```python
from build123d import *

# Parameters (mm, degrees)
F0_W     = 14.0914916992
F0_H     = 13.3883208036
F0_H_2   = 4.0725544095
F1_DEPTH = 25.4
F2_R     = 5.08


with BuildPart() as f1:
    # F0 (on Top) → F1 (new body)
    with BuildSketch(Plane.XY):
        Polygon((-14.0914916992, 52.0800277591), (-14.0914916992, 65.4683485627), (0, 65.4683485627), (0, 52.0800277591), (26.658244431, 52.0800277591), (26.658244431, 110.8265519142), (-39.2834246159, 110.8265519142), (-39.2834246159, 52.0800277591), align=None)
        with Locations((-7.0457458496, 58.7741881609)):
            Rectangle(F0_W, F0_H)
        with Locations((-7.0457458496, 50.0437505543)):
            Rectangle(F0_W, F0_H_2)
    extrude(amount=F1_DEPTH)

    # F2
    f2_edges = [f1.edges().sort_by_distance(p)[0] for p in [
        (26.658244, 81.45329, 25.4),
        (26.658244, 81.45329, 0),
        (-39.283425, 81.45329, 25.4),
        (-6.31259, 110.826552, 25.4),
    ]]
    fillet(f2_edges, radius=F2_R)


solid = f1.part
```
Build history of the part. All positions in model axes, mm. A direction names the side the tool comes from. Coordinates: 2 decimals unless noted, no trailing zeros. Order: outer loops, then holes, each group sorted by start corner. A loop starts at its lowest first (then second) coordinate and runs counter-clockwise, first axis right, second up. Notation, with made-up numbers: M 2,16 L 24,16 A25 ccw 24,33 Z; hole C 66,-21.5 d11. An arc over 180 degrees is marked long. One line per question, with ' | ' between items. Start each with the question number.
1. Cut at B-B (x = -28). Write the cut outline in (y, z), plus the area to 3 significant figures.
2. Cut at A-A (z = 18.75). Write the cut outline in (x, y).
3. Tool access for faces 1 (the face through (-14.091, 50, 13)), 2 (the face through (-6, 110.827, 10)), 3 (the face through (0, 50, 13)): list every direction of +Z, -Z, +X, -X, +Y, -Y with a clear straight run to the whole face (end or side of a thin tool).
4. Flat gauge pins, fed straight in: P1, Ø12.5, axis at x = 17.5, z = 18.5, coming from the -Y side; P2, Ø12, axis at y = 102.5, z = 22.5, coming from the +X side; P3, Ø3.5, axis at y = 49.5, z = 15.5, coming from the -X side; P4, Ø1.2, axis at y = 50, z = 12.5, coming from the +X side. Where does each tip first touch, or does it go through?
5. Wall check: line 1 along Y through (x, z) = (-29.5, 15.5); line 2 along X through (y, z) = (58, 21.5); line 3 along Z through (x, y) = (24.5, 87). Give the ranges that are in metal, low to high. Write a range as [from, to].
The answers:
1) outline: M 52.08,0 L 110.83,0 L 110.83,20.32 A5.08 ccw 105.75,25.4 L 52.08,25.4 Z | area: 1,490 mm2
2) outline: M -39.28,52.08 L -14.09,52.08 L -14.09,48.01 L 0,48.01 L 0,52.08 L 26.66,52.08 L 26.66,110.83 L -39.28,110.83 Z
3) face 1: +Z, -Z, -X, -Y | face 2: +Z, -Z, +X, -X, +Y | face 3: +Z, -Z, +X, -Y
4) P1: stops at y = 52.08 | P2: stops at x = 26.66 | P3: stops at x = -14.09 | P4: stops at x = 0
5) line 1: y = [52.08, 110.83] | line 2: x = [-39.14, 26.52] | line 3: z = [0.92, 24.48]
